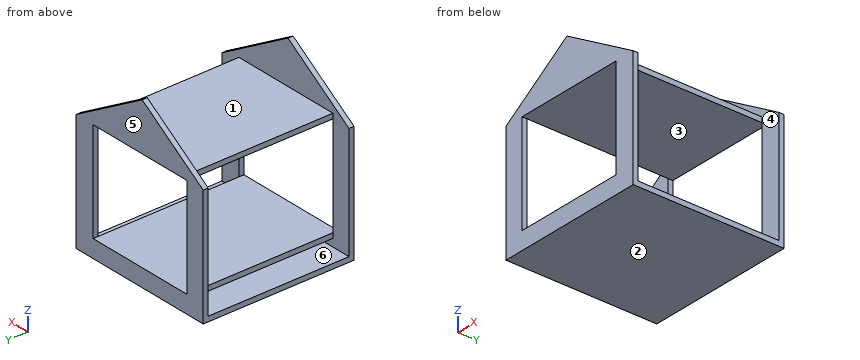
from build123d import *

# Parameters (mm, degrees)
F0_W     = 10.2729936957
F0_H     = 50.8
F0_W_2   = 9.6539677948
F1_DEPTH = 76.2
F2_T     = 2.54


# Not quite as in the source:
# - a shell that OpenCascade refuses in one call is made with other operations: the cavity is built on its own and cut out


with BuildPart() as f1:
    # F0 (on Front) → F1 (new body)
    with BuildSketch(Plane.XZ):
        Polygon((-4.9094697461, 50.2964220941), (-41.4324142039, 26.1541400105), (-31.7784464091, 26.1541400105), (24.4945921004, 26.1541400105), (34.7675857961, 26.1541400105), align=None)
        with Locations((29.6310889482, 0.7541400105)):
            Rectangle(F0_W, F0_H)
        with Locations((-36.6054303065, 0.7541400105)):
            Rectangle(F0_W_2, F0_H)
        Polygon((-31.7784464091, -24.6458599895), (-41.4324142039, -24.6458599895), (-41.4324142039, -33.582534641), (34.7675857961, -33.582534641), (34.7675857961, -24.6458599895), (24.4945921004, -24.6458599895), align=None)
    extrude(amount=F1_DEPTH)

    # F2: shell of thickness 2.54, made by hand


with BuildPart() as f2_core1:
    # F2_t2: copy of F1
    add(f1.part)

    # the walls: a layer under each face that stays
    f2_faces = [f2_core1.faces().sort_by_distance(p)[0] for p in [
        (-3.3324142039, -38.1, -33.582534641),
        (-3.6419271544, -38.1, 26.1541400105),
        (-3.6419271544, -38.1, -24.6458599895),
        (-3.3324142039, 0, 36.3165959716),
        (-3.3324142039, -76.2, 36.3165959716),
    ]]
    thicken(f2_faces, amount=-F2_T, mode=Mode.SUBTRACT)


with BuildPart() as f1_1:
    add(f1.part)

    # what is left inside the walls is the cavity
    f2_cavity = [f2_core1.part.solids().sort_by_distance(p)[0] for p in [
        (-3.332414, -49.953333, -31.017135),
    ]]
    add(f2_cavity, mode=Mode.SUBTRACT)


solid = f1_1.part
Verification items for the finished model (mm, model axes). Face numbers are marked on the shaded views. A direction names the side the tool comes from. Coordinates: 2 decimals unless noted, no trailing zeros. Order: outer loops, then holes, each group sorted by start corner. A loop starts at its lowest first (then second) coordinate and runs counter-clockwise, first axis right, second up.
Item 1: Material ranges on L1, parallel to Z at x = 0.5, y = -9.5; L2, parallel to Y at x = -27, z = 35.5; L3, parallel to Z at x = 31, y = -35, recorded low to high.
Filled in:
L1: z = -33.58 to -31.04, -27.19 to -24.65, 26.15 to 28.69
L2: y = -76.2 to -73.66, -2.54 to 0
L3: z = -33.58 to -31.04
Item 2: Release check for a two-part mould opening along Y. For the marked faces 3, 4, 5 and 6 record: +Y half, -Y half, draft (parallel to the pull), parting line (faces both ways), or undercut.
Filled in:
face 3: draft
face 4: undercut
face 5: +Y half
face 6: undercut
Item 3: Depth check by flat-ended pin: pin 1 (2 mm diameter, centred on y = -35.5, z = 27, fed in from -X); pin 2 (3 mm diameter, centred on x = 13.5, z = 24.5, fed in from +Y); pin 3 (2 mm diameter, centred on y = -25, z = -26.5, fed in from +X); pin 4 (10 mm diameter, centred on x = -33.5, y = -33, fed in from +Z). Enter the tip coordinate at first touch or a pass-through.
Filled in:
pin 1: stops at x = -31.78
pin 2: passes through
pin 3: stops at x = 24.49
pin 4: stops at z = 28.69
Item 4: Access from +Z, -Z, +X, -X, +Y, -Y to the whole of each face (thin tool, end or side, straight path). Record for the marked faces 1 and 2.
Filled in:
face 1: +Z, +X, -X
face 2: -Z, +X, -X, +Y, -Y
Item 5: Section check D-D, the plane x = -18. Enter the section's corners in (y, z), then the cut area to 3 significant figures.
Filled in:
outline: (-76.2, -33.58) - (0, -33.58) - (0, -24.65) - (-76.2, -24.65) - close; (-76.2, 26.15) - (0, 26.15) - (0, 41.64) - (-2.54, 41.64) - (-2.54, 28.69) - (-73.66, 28.69) - (-73.66, 41.64) - (-76.2, 41.64) - close; hole (-73.66, -31.04) - (-2.54, -31.04) - (-2.54, -27.19) - (-73.66, -27.19) - close
area: 666 mm2
Item 6: Section check B-B, the plane x = -10. Enter the section's corners in (y, z), then the cut area to 3 significant figures.
Filled in:
outline: (-76.2, -33.58) - (0, -33.58) - (0, -24.65) - (-76.2, -24.65) - close; (-76.2, 26.15) - (0, 26.15) - (0, 46.93) - (-2.54, 46.93) - (-2.54, 28.69) - (-73.66, 28.69) - (-73.66, 46.93) - (-76.2, 46.93) - close; hole (-73.66, -31.04) - (-2.54, -31.04) - (-2.54, -27.19) - (-73.66, -27.19) - close
area: 693 mm2
Item 7: Section check A-A, the plane z = -11.5. Enter the section's corners in (x, y).
Filled in:
outline: (-41.43, -76.2) - (-31.78, -76.2) - (-31.78, -73.66) - (-41.43, -73.66) - close; (-41.43, -2.54) - (-31.78, -2.54) - (-31.78, 0) - (-41.43, 0) - close; (24.49, -76.2) - (34.77, -76.2) - (34.77, -73.66) - (24.49, -73.66) - close; (24.49, -2.54) - (34.77, -2.54) - (34.77, 0) - (24.49, 0) - close
Item 8: Section check C-C, the plane y = -35.5. Enter the section's corners in (x, z).
Filled in:
outline: (-41.43, -33.58) - (34.77, -33.58) - (34.77, -31.04) - (-41.43, -31.04) - close; (-31.78, -27.19) - (24.49, -27.19) - (24.49, -24.65) - (-31.78, -24.65) - close; (-31.78, 26.15) - (24.49, 26.15) - (24.49, 28.69) - (-31.78, 28.69) - close
